Input: part model. Units: mm. Frame: model coordinates. Give positions to 0.01 mm unless a question says otherwise; leave off trailing zeros. Write each loop counter-clockwise with the first axis right and the second up, starting at its lowest first coordinate (ties: lowest second). Pieces come first, ordered by that corner, then holes. Notation, with made-up numbers: (4.5, -31.5) - (13.5, -31.5) arc R25 ccw to (13.5, -6.5) - close; hole circle Ø11 at (16, 64). An arc over 180 degrees is marked (long way). Use a Markdown table: item, result. Add a question column.
1. Section query D-D, the plane x = 180. Return loops of the section in (y, z).
2. Pin query (flat end, axial travel): pin 1 (10 mm diameter, centred on x = -11, z = 24, fed in from -Y). Return the tip coordinate at first contact, or that it passes through.
3. Material intervals for probe 1 along Y at (x, z) = (0, 1); probe 2 along Z at (x, y) = (-57, 171), sorted ascending.
4. Section query A-A, the plane y = 0. Return loops of the section in (x, z).
5. Section query C-C, the plane y = -112.5. Return loops of the section in (x, z).
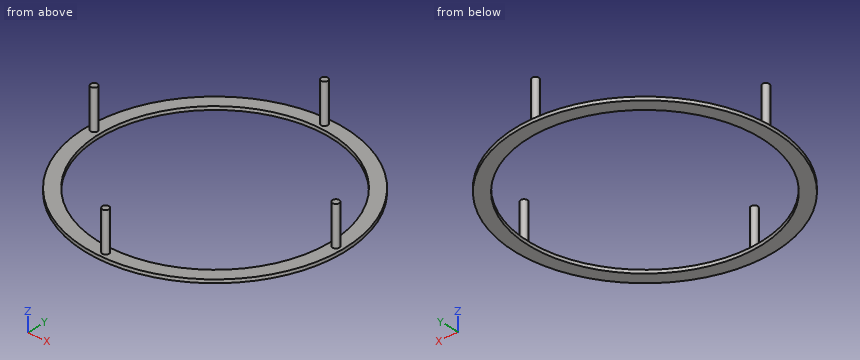
```python
from build123d import *

# Parameters (mm, degrees)
SKETCH_1_R      = 190
SKETCH_1_R_2    = 170
EXTRUDE_2_DEPTH = 5
SKETCH_2_R      = 5
EXTRUDE_3_DEPTH = 58


with BuildPart() as part:
    # 草图1 → 凸台-拉伸2 (new body)
    with BuildSketch(Plane.XY):
        Circle(SKETCH_1_R)
        Circle(SKETCH_1_R_2, mode=Mode.SUBTRACT)
    extrude(amount=EXTRUDE_2_DEPTH)

    # 草图2 → 凸台-拉伸3 (add)
    with BuildSketch(Plane.XY.offset(5)):
        with Locations(Location((0, 180, 0), (0, 0, 180))):
            Circle(SKETCH_2_R)
        with Locations(Location((-180, 0, 0), (0, 0, 180))):
            Circle(SKETCH_2_R)
        with Locations(Location((0, -180, 0), (0, 0, 180))):
            Circle(SKETCH_2_R)
        with Locations(Location((180, 0, 0), (0, 0, 180))):
            Circle(SKETCH_2_R)
    extrude(amount=EXTRUDE_3_DEPTH)


solid = part.part
```
Result sheet:
| question | item | result |
|---|---|---|
| 1 | outline | (-60.83, 0) - (60.83, 0) - (60.83, 5) - (5, 5) - (5, 63) - (-5, 63) - (-5, 5) - (-60.83, 5) - close |
| 2 | pin 1 | passes through |
| 3 | probe 1 | y = -190 to -170, 170 to 190 |
| 3 | probe 2 | z = 0 to 5 |
| 4 | outline | (-190, 0) - (-170, 0) - (-170, 5) - (-175, 5) - (-175, 63) - (-185, 63) - (-185, 5) - (-190, 5) - close; (170, 0) - (190, 0) - (190, 5) - (185, 5) - (185, 63) - (175, 63) - (175, 5) - (170, 5) - close |
| 5 | outline | (-153.11, 0) - (-127.45, 0) - (-127.45, 5) - (-153.11, 5) - close; (127.45, 0) - (153.11, 0) - (153.11, 5) - (127.45, 5) - close |
